Geometry: final body of the model. Coordinates: model frame, mm. Give positions to 0.01 mm unless a question says otherwise; leave off trailing zeros. Write each loop counter-clockwise with the first axis right and the second up, starting at its lowest first coordinate (ties: lowest second). Pieces come first, ordered by that corner, then holes. Notation, with made-up numbers: (29.25, 58.5) - (66.25, 58.5) arc R13 cw to (66.25, 77.5) - close; hole circle Ø9 at (9.5, 14). An arc over 180 degrees is marked (long way). Use CSV: the item, a comma, the result in double quotes. Start each with the question number.
(1) Section B-B on y = 8. Output: boundary loops of the cut face in (x, z), and give its area (3 significant figures).
(2) Draft query along X for faces 1 (the flat face through (-13, 5, 0)), 2 (the cylindrical face through (-1.57, 9.35, -20.79)), 3 (the cylindrical face through (-23.43, 1.65, -20.79)). Return one class per face: released by +X, released by -X, zero draft, split by the parting line, or undercut.
(3) Section C-C on x = -3.75. Output: boundary loops of the cut face in (y, z), and give its area (3 significant figures).
(4) First-contact query: pin 1 Ø3 at (x, z) = (-21.5, -13) entering from -Y. Flat tip, straight axial feed; report the tip coordinate or a pass-through.
(5) Line query: probe 1 along Y at (x, z) = (-5.25, -28); probe 2 along X at (y, z) = (5.25, -37); probe 3 along X at (y, z) = (8, -30). Output: solid intervals per line, ascending. Write a range as [from, to].
from build123d import *

# Parameters (mm, degrees)
SCHIZZO1_W                   = 25
SCHIZZO1_H                   = 41
ESTRUSIONE_ESTRUSIONE1_DEPTH = 11
RACCORDO1_R                  = 5.5


with BuildPart() as part:
    # Schizzo1 → Estrusione-Estrusione1 (new body)
    with BuildSketch(Plane(origin=(0, 0, 0), x_dir=(1, 0, 0), z_dir=(0, 1, 0))):
        with Locations((-12.5, 20.5)):
            Rectangle(SCHIZZO1_W, SCHIZZO1_H)
    extrude(amount=ESTRUSIONE_ESTRUSIONE1_DEPTH)

    # Raccordo1
    raccordo1_edges = [part.edges().sort_by_distance(p)[0] for p in [
        (-25, 11, -20.5),
        (-25, 0, -20.5),
        (0, 0, -20.5),
        (0, 11, -20.5),
    ]]
    fillet(raccordo1_edges, radius=RACCORDO1_R - 0.0001)  # a hair under: the kernel refuses the full size


solid = part.part
Check values:
1,outline,"(-24.4, -41) - (-0.6, -41) - (-0.6, 0) - (-24.4, 0) - close"
1,area,"976 mm²"
2,face 1,"zero draft"
2,face 2,"released by +X"
2,face 3,"released by -X"
3,outline,"(0.29, -41) - (10.71, -41) - (10.71, 0) - (0.29, 0) - close"
3,area,"428 mm²"
4,pin 1,"stops at y = 0.02"
5,probe 1,"y = [0.01, 10.99]"
5,probe 2,"x = [-24.99, -0.01]"
5,probe 3,"x = [-24.4, -0.6]"
